from build123d import *

# Parameters (mm, degrees)
EXTRUDE_1_DEPTH     = 8.25
CUT_EXTRUDE_1_DEPTH = 5
SKETCH_4_R          = 0.5
SKETCH_4_R_2        = 0.517195783
CUT_EXTRUDE_2_DEPTH = 5
CUT_EXTRUDE_3_DEPTH = 0.1
SKETCH_6_R          = 0.157252924
CUT_EXTRUDE_4_DEPTH = 0.1
CUT_EXTRUDE_5_DEPTH = 0.1
CUT_EXTRUDE_6_DEPTH = 0.1
CUT_EXTRUDE_7_DEPTH = 10


with BuildPart() as part:
    # 草图1 → 凸台-拉伸1 (new body)
    with BuildSketch(Plane.XY):
        with BuildLine():
            Line((-18.031435036, 37.379055707), (38.668564964, 37.379055707))
            ThreePointArc((38.668564964, 37.379055707), (45.739632776, 34.450123519), (48.668564964, 27.379055707))
            Line((48.668564964, 27.379055707), (48.668564964, -112.520944293))
            ThreePointArc((48.668564964, -112.520944293), (45.739632776, -119.592012105), (38.668564964, -122.520944293))
            Line((38.668564964, -122.520944293), (-18.031435036, -122.520944293))
            ThreePointArc((-18.031435036, -122.520944293), (-25.102502847, -119.592012105), (-28.031435036, -112.520944293))
            Line((-28.031435036, -112.520944293), (-28.031435036, 27.379055707))
            ThreePointArc((-28.031435036, 27.379055707), (-25.102502847, 34.450123519), (-18.031435036, 37.379055707))
        make_face()
    extrude(amount=EXTRUDE_1_DEPTH)

    # 草图2 → 切除-拉伸1 (cut)
    with BuildSketch(Plane.XZ.offset(122.520944293)):
        with BuildLine():
            Line((6.427510461, 6.234889493), (14.427510461, 6.234889493))
            ThreePointArc((14.427510461, 6.234889493), (15.927510461, 4.734889493), (14.427510461, 3.234889493))
            Line((14.427510461, 3.234889493), (6.427510461, 3.234889493))
            ThreePointArc((6.427510461, 3.234889493), (4.927510461, 4.734889493), (6.427510461, 6.234889493))
        make_face()
    extrude(amount=-CUT_EXTRUDE_1_DEPTH, mode=Mode.SUBTRACT)

    # 草图4 → 切除-拉伸2 (cut)
    with BuildSketch(Plane.XZ.offset(122.520944293)):
        with Locations(Location((2, 4.719775151, 0), (0, 0, 270))):
            Circle(SKETCH_4_R)
        with Locations(Location((0, 4.71977515, 0), (0, 0, 270))):
            Circle(SKETCH_4_R)
        with Locations(Location((-2, 4.71977515, 0), (0, 0, 270))):
            Circle(SKETCH_4_R)
        with Locations(Location((-4, 4.71977515, 0), (0, 0, 270))):
            Circle(SKETCH_4_R)
        with Locations(Location((18, 4.71977515, 0), (0, 0, 270))):
            Circle(SKETCH_4_R_2)
        with Locations(Location((20, 4.71977515, 0), (0, 0, 270))):
            Circle(SKETCH_4_R)
        with Locations(Location((22, 4.71977515, 0), (0, 0, 270))):
            Circle(SKETCH_4_R)
        with Locations(Location((24, 4.71977515, 0), (0, 0, 270))):
            Circle(SKETCH_4_R)
        with Locations(Location((26, 4.71977515, 0), (0, 0, 270))):
            Circle(SKETCH_4_R)
        with Locations(Location((28, 4.71977515, 0), (0, 0, 270))):
            Circle(SKETCH_4_R)
    extrude(amount=-CUT_EXTRUDE_2_DEPTH, mode=Mode.SUBTRACT)

    # 草图5 → 切除-拉伸3 (cut)
    with BuildSketch(Plane(origin=(48.668564964, 0, 0), x_dir=(0, 0, -1), z_dir=(1, 0, 0))):
        with BuildLine():
            Line((-2.555232712, 3.731296592), (-2.555232712, -12.268703408))
            ThreePointArc((-2.555232712, -12.268703408), (-4.055232712, -13.768703408), (-5.555232712, -12.268703408))
            Line((-5.555232712, -12.268703408), (-5.555232712, 3.731296592))
            ThreePointArc((-5.555232712, 3.731296592), (-4.055232712, 5.231296592), (-2.555232712, 3.731296592))
        make_face()
    extrude(amount=-CUT_EXTRUDE_3_DEPTH, mode=Mode.SUBTRACT)

    # 草图6 → 切除-拉伸4 (cut)
    with BuildSketch(Plane.ZY.offset(28.031435036)):
        with Locations(Location((4.361987168, 13.879950774, 0), (0, 0, 270))):
            Circle(SKETCH_6_R)
        with BuildLine():
            Line((5.5, -11.5), (5.5, -22.5))
            ThreePointArc((5.5, -22.5), (4, -24), (2.5, -22.5))
            Line((2.5, -22.5), (2.5, -11.5))
            ThreePointArc((2.5, -11.5), (4, -10), (5.5, -11.5))
        make_face()
        with BuildLine():
            Line((5.5, 5.5), (5.5, -5.5))
            ThreePointArc((5.5, -5.5), (4, -7), (2.5, -5.5))
            Line((2.5, -5.5), (2.5, 5.5))
            ThreePointArc((2.5, 5.5), (4, 7), (5.5, 5.5))
        make_face()
    extrude(amount=-CUT_EXTRUDE_4_DEPTH, mode=Mode.SUBTRACT)

    # 草图9 → 切除-拉伸5 (cut)
    with BuildSketch(Plane.ZY.offset(28.031435036)):
        with BuildLine():
            Line((5.5, 18), (5.5, 12))
            ThreePointArc((5.5, 12), (4, 10.5), (2.5, 12))
            Line((2.5, 12), (2.5, 18))
            ThreePointArc((2.5, 18), (4, 19.5), (5.5, 18))
        make_face()
    extrude(amount=-CUT_EXTRUDE_5_DEPTH, mode=Mode.SUBTRACT)

    # 草图10 → 切除-拉伸6 (cut)
    with BuildSketch(Plane(origin=(0, 0, 0), x_dir=(-1, 0, 0), z_dir=(0, 0, -1))):
        with BuildLine():
            Line((-31.830127614, 25.033557379), (-7.830127614, 25.033557379))
            ThreePointArc((-7.830127614, 25.033557379), (-2.173273364, 22.690411628), (0.169872386, 17.033557379))
            Line((0.169872386, 17.033557379), (0.169872386, -6.966442621))
            ThreePointArc((0.169872386, -6.966442621), (-2.173273364, -12.623296871), (-7.830127614, -14.966442621))
            Line((-7.830127614, -14.966442621), (-31.830127614, -14.966442621))
            ThreePointArc((-31.830127614, -14.966442621), (-37.486981863, -12.623296871), (-39.830127614, -6.966442621))
            Line((-39.830127614, -6.966442621), (-39.830127614, 17.033557379))
            ThreePointArc((-39.830127614, 17.033557379), (-37.486981863, 22.690411628), (-31.830127614, 25.033557379))
        make_face()
    extrude(amount=-CUT_EXTRUDE_6_DEPTH, mode=Mode.SUBTRACT)

    # 草图11 → 切除-拉伸7 (cut)
    with BuildSketch(Plane.ZY.offset(28.031435036)):
        with BuildLine():
            Line((5.5, -40), (5.5, -56))
            ThreePointArc((5.5, -56), (4, -57.5), (2.5, -56))
            Line((2.5, -56), (2.5, -40))
            ThreePointArc((2.5, -40), (4, -38.5), (5.5, -40))
        make_face()
    extrude(amount=-CUT_EXTRUDE_7_DEPTH, mode=Mode.SUBTRACT)


solid = part.part
Build history of the part. All positions in model axes, mm. A direction names the side the tool comes from. Coordinates: 2 decimals unless noted, no trailing zeros. Write item = value, one per line. Start each with the question number.
1) Wall check: line 1 along Y through (x, z) = (22, 4.25); line 2 along Y through (x, z) = (-21, 4.5); line 3 along X through (y, z) = (19, 3.25). Give the ranges that are in metal, low to high. Write a range as from..to.
2) Flat gauge pins, fed straight in: pin 1 Ø5.5 at (x, y) = (12, -119) entering from -Z; pin 2 Ø2.5 at (y, z) = (-45, 4) entering from -X; pin 3 Ø0.5 at (x, z) = (24, 4.5) entering from -Y; pin 4 Ø12 at (x, y) = (15, 10.5) entering from -Z. Where does each tip first touch, or does it go through?
3) Two-plate mould, pull along Y, no slides. Class faces 1 (the face through (-23, -48, 5.5)), 2 (the face through (10, 37.379, 4)), 3 (the face through (-28.031, -44, 2)), 4 (the face through (-23, -48, 2.5)): pulls with the +Y half, pulls with the -Y half, needs draft (parallel to the pull), parting line crosses it, or undercut.
4) 3-axis set-ups, long thin cutter, end or side, ignore diameter. For faces 5 (the face through (10, -120, 3.235)), 6 (the face through (-23.1, -38.5, 4)): which of +Z, -Z, +X, -X, +Y, -Y reach the whole face in a straight line?
From the geometry:
q1.line_1 = -117.52..37.38
q1.line_2 = -122.07..-57.41, -38.59..36.93
q1.line_3 = -27.93..48.67
q2.pin_1 = 0
q2.pin_2 = -18.03
q2.pin_3 = -117.52
q2.pin_4 = 0.1
q3.face_1 = undercut
q3.face_2 = pulls with the +Y half
q3.face_3 = needs draft
q3.face_4 = undercut
q4.face_5 = -Y
q4.face_6 = -X
